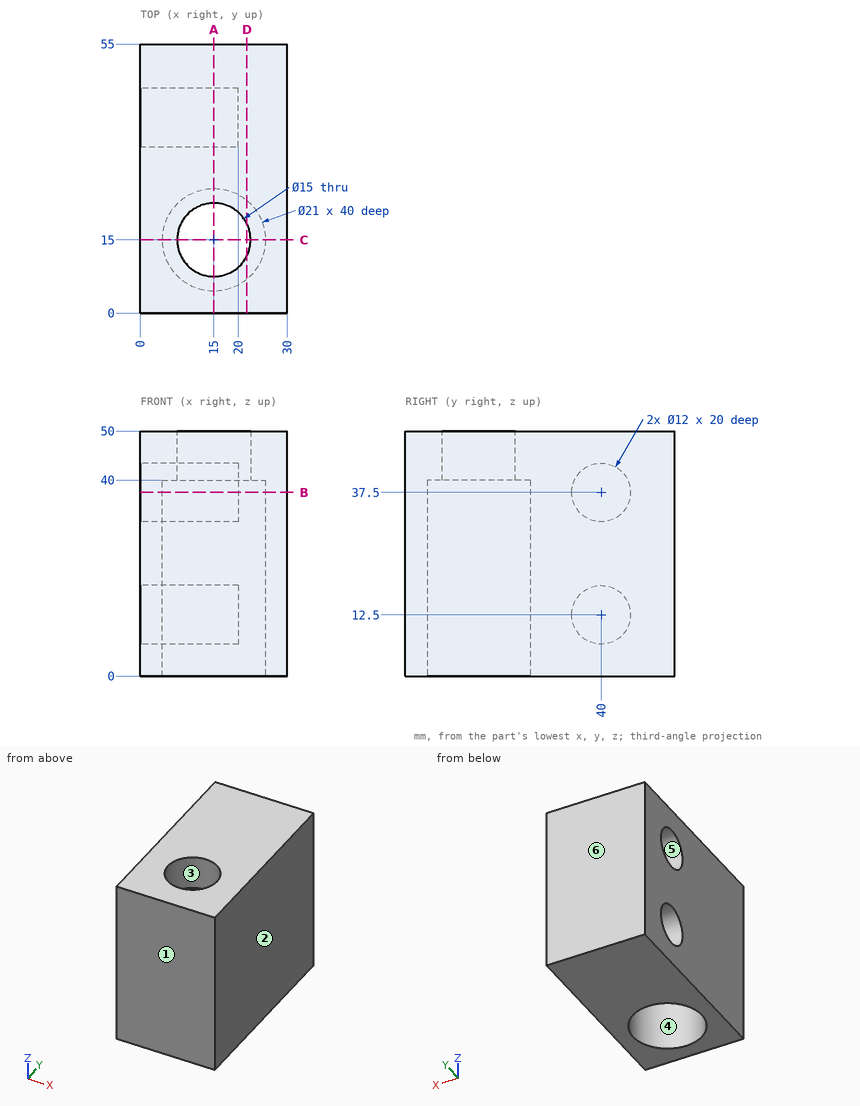
Could you check a few things on this drawing? It's one solid part, dimensions in mm from its lowest x, y, z. A direction names the side the tool comes from. Give positions to 0.01 mm unless a question says otherwise; leave off trailing zeros. Order: outer loops, then holes, each group sorted by start corner. A loop starts at its lowest first (then second) coordinate and runs counter-clockwise, first axis right, second up. Notation, with made-up numbers: (41, -29) - (81, -29) arc R22 cw to (81, 6) - close; hole circle Ø4 at (-14.75, 13.25). An arc over 180 degrees is marked (long way). One line per question, with ' | ' between items. Start each with the question number.
Item 1: I want a section at A-A on x = 15. Write out the boundary of the cut face in (y, z).
Item 2: For the marked faces 5 and 6, which set-ups out of +Z, -Z, +X, -X, +Y, -Y let a thin tool reach every point of the face, with its end or its side?
Item 3: Thinking about a two-plate mould opening in Y: for the marked faces 1, 2, 3 and 4, which applies, pulls with the +Y half, pulls with the -Y half, needs draft (parallel to the pull), parting line crosses it, or undercut?
Item 4: I want a section at D-D on x = 21.75. Write out the boundary of the cut face in (y, z), then the cut area to 3 significant figures.
Item 5: I want a section at C-C on y = 15. Write out the boundary of the cut face in (x, z).
Item 6: I'm going to push flat-ended pins straight in: pin 1 Ø10.5 at (x, y) = (18, 17.5) entering from -Z; pin 2 Ø11 at (y, z) = (40, 37.5) entering from -X. Where does each tip first touch, or does it pass through?
Item 7: I want a section at B-B on z = 37.5. Write out the boundary of the cut face in (x, y), then the cut area to 3 significant figures.
Item 8: I need wall thicknesses on probe 1 along Z at (x, y) = (11.25, 40); probe 2 along Y at (x, z) = (15, 31); probe 3 along Y at (x, z) = (15, 46.75). Which ranges of each line are inside material? Lowest first, please. Write a range as [from, to].
Verdict:
1) outline: (0, 0) - (4.5, 0) - (4.5, 40) - (7.5, 40) - (7.5, 50) - (0, 50) - close; (22.5, 40) - (25.5, 40) - (25.5, 0) - (55, 0) - (55, 50) - (22.5, 50) - close; hole circle Ø12 at (40, 12.5); hole circle Ø12 at (40, 37.5)
2) face 5: -X | face 6: +Z, -Z, +X, -X, +Y
3) face 1: pulls with the -Y half | face 2: needs draft | face 3: undercut | face 4: undercut
4) outline: (0, 0) - (6.96, 0) - (6.96, 40) - (11.73, 40) - (11.73, 50) - (0, 50) - close; (18.27, 40) - (23.04, 40) - (23.04, 0) - (55, 0) - (55, 50) - (18.27, 50) - close | area: 2,040 mm^2
5) outline: (0, 0) - (4.5, 0) - (4.5, 40) - (7.5, 40) - (7.5, 50) - (0, 50) - close; (22.5, 40) - (25.5, 40) - (25.5, 0) - (30, 0) - (30, 50) - (22.5, 50) - close
6) pin 1: z = 40 | pin 2: x = 20
7) outline: (0, 0) - (30, 0) - (30, 55) - (0, 55) - (0, 46) - (20, 46) - (20, 34) - (0, 34) - close; hole circle Ø21 at (15, 15) | area: 1,060 mm^2
8) probe 1: [0, 6.5], [18.5, 31.5], [43.5, 50] | probe 2: [0, 4.5], [25.5, 55] | probe 3: [0, 7.5], [22.5, 55]
